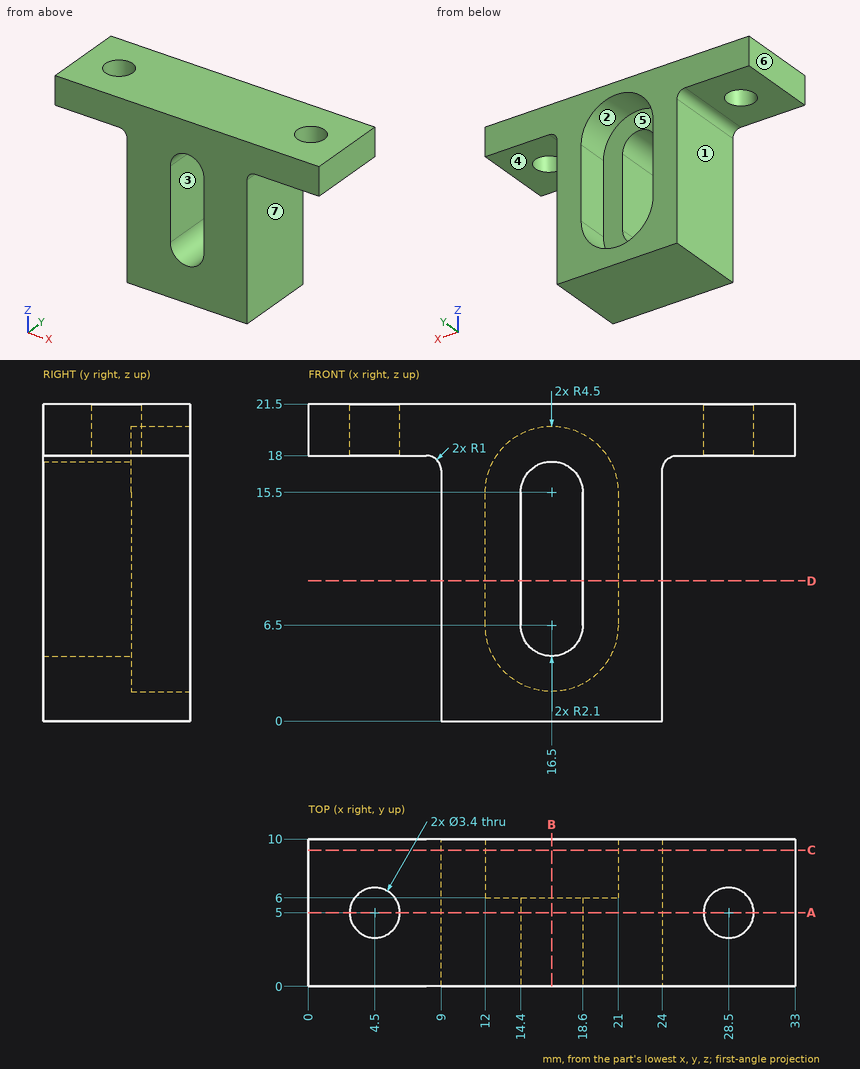
Answer from the drawing. Dimensions are ordinates in mm from the lowest x, y and z of the part. A direction names the side the tool comes from. Round coordinates to 2 decimals unless told otherwise and drop trailing zeros. Write each loop counter-clockwise with the first axis right and the second up, starting at its lowest first coordinate (ties: lowest second). Pieces come first, ordered by that corner, then holes. Notation, with made-up numbers: (-36, 29.5) -> (16, 29.5) arc R21 ccw to (16, 51.5) -> close; hole circle Ø8 at (9, 89). An arc over 180 degrees is marked (long way). Answer in a Markdown table with one row per item. Add a question column.
1) Determine the mould class of the marked faces 4, 5, 6 and 7 for opening direction X: pulls with the +X half, pulls with the -X half, needs draft (parallel to the pull), parting line crosses it, or undercut.
2) Find section C-C, the plane y = 9.25. Determine the outline of the cut face in (x, z).
3) Which of the six approach directions +Z, -Z, +X, -X, +Y, -Y give full straight-line access (tool end or side, diameter ignored) to the marked faces 1, 2 and 3?
4) Find section A-A, the plane y = 5. Determine the outline of the cut face in (x, z).
5) Consider line 1 (X direction, y = 7.5, z = 15.75); line 2 (Y direction, x = 4.5, z = 20.4); line 3 (X direction, y = 6, z = 20.5). Determine where each line is inside the solid, lowest interval first.
6) Find section B-B, the plane x = 16.5. Determine the outline of the cut face in (y, z), and give its area (3 significant figures).
7) Find section D-D, the plane z = 9.5. Determine the outline of the cut face in (x, y), and give its area (3 significant figures).
8) Given P1, Ø2, axis at y = 8.5, z = 11, coming from the -X side; P2, Ø6, axis at x = 17, z = 7, coming from the +Y side; P3, Ø2.5, axis at x = 28.5, y = 6, coming from the -Z side; P4, Ø4, axis at x = 5.5, z = 14, coming from the -Y side, each flat-ended and moving along its own axis, determine where each tip first touches the part or whether it passes through.
Findings below:
| question | item | result |
|---|---|---|
| 1 | face 4 | needs draft |
| 1 | face 5 | undercut |
| 1 | face 6 | pulls with the -X half |
| 1 | face 7 | pulls with the +X half |
| 2 | outline | (0, 18) -> (8, 18) arc R1 cw to (9, 17) -> (9, 0) -> (24, 0) -> (24, 17) arc R1 cw to (25, 18) -> (33, 18) -> (33, 21.5) -> (0, 21.5) -> close; hole (12, 6.5) arc R4.5 ccw to (21, 6.5) -> (21, 15.5) arc R4.5 ccw to (12, 15.5) -> close |
| 3 | face 1 | -Z, -X, +Y, -Y |
| 3 | face 2 | +Y |
| 3 | face 3 | +Y, -Y |
| 4 | outline | (0, 18) -> (2.8, 18) -> (2.8, 21.5) -> (0, 21.5) -> close; (6.2, 18) -> (8, 18) arc R1 cw to (9, 17) -> (9, 0) -> (24, 0) -> (24, 17) arc R1 cw to (25, 18) -> (26.8, 18) -> (26.8, 21.5) -> (6.2, 21.5) -> close; (30.2, 18) -> (33, 18) -> (33, 21.5) -> (30.2, 21.5) -> close; hole (14.4, 6.5) arc R2.1 ccw to (18.6, 6.5) -> (18.6, 15.5) arc R2.1 ccw to (14.4, 15.5) -> close |
| 5 | line 1 | 9 to 12.01, 20.99 to 24 |
| 5 | line 2 | 0 to 3.3, 6.7 to 10 |
| 5 | line 3 | 0 to 3.13, 5.87 to 27.13, 29.87 to 33 |
| 6 | outline | (0, 0) -> (10, 0) -> (10, 2) -> (6, 2) -> (6, 4.4) -> (0, 4.4) -> close; (0, 17.6) -> (6, 17.6) -> (6, 20) -> (10, 20) -> (10, 21.5) -> (0, 21.5) -> close |
| 6 | area | 63.8 mm² |
| 7 | outline | (9, 0) -> (14.4, 0) -> (14.4, 6) -> (12, 6) -> (12, 10) -> (9, 10) -> close; (18.6, 0) -> (24, 0) -> (24, 10) -> (21, 10) -> (21, 6) -> (18.6, 6) -> close |
| 7 | area | 88.8 mm² |
| 8 | P1 | x = 9 |
| 8 | P2 | y = 6 |
| 8 | P3 | z = 18 |
| 8 | P4 | through |
